from build123d import *

# Parameters (mm, degrees)
SKETCH1_R           = 2.95
SKETCH1_R_2         = 20
SKETCH1_R_3         = 18.5
BOSS_EXTRUDE1_DEPTH = 6
CUT_EXTRUDE2_DEPTH  = 76.689323992
SKETCH4_W           = 6.2
SKETCH4_H           = 2.2
CUT_EXTRUDE3_DEPTH  = 76.689323992


with BuildPart() as part:
    # Sketch1 → Boss-Extrude1 (new body)
    with BuildSketch(Plane.XY):
        Polygon((-32.5, 7.5), (-32.5, -22), (32.5, -22), (32.5, 7.5), (49.675685802, 7.5), (49.675685802, 56.790844389), (-49.675685802, 56.790844389), (-49.675685802, 7.5), align=None)
        Circle(SKETCH1_R, mode=Mode.SUBTRACT)
        with Locations((26.675685802, 31.790844389)):
            Circle(SKETCH1_R_2, mode=Mode.SUBTRACT)
        with Locations((-26.675685802, 31.790844389)):
            Circle(SKETCH1_R_3, mode=Mode.SUBTRACT)
    extrude(amount=BOSS_EXTRUDE1_DEPTH)

    # Sketch3 → Cut-Extrude2 (cut, through all)
    with BuildSketch(Plane.XY.offset(6)):
        Polygon((-12.3, -22), (-7.7, -22), (-7.7, -17), (-5.4, -17), (-5.4, -14), (-7.7, -14), (-7.7, -10), (-12.3, -10), (-12.3, -14), (-14.6, -14), (-14.6, -17), (-12.3, -17), align=None)
        Polygon((7.7, -14), (7.7, -10), (12.3, -10), (12.3, -14), (14.6, -14), (14.6, -17), (12.3, -17), (12.3, -22), (7.7, -22), (7.7, -17), (5.4, -17), (5.4, -14), align=None)
    extrude(amount=-CUT_EXTRUDE2_DEPTH, mode=Mode.SUBTRACT)

    # Sketch4 → Cut-Extrude3 (cut, through all)
    with BuildSketch(Plane.XY.offset(6)):
        with Locations((0, 52.690844389)):
            Rectangle(SKETCH4_W, SKETCH4_H)
        with Locations((44, 52.690844389)):
            Rectangle(SKETCH4_W, SKETCH4_H)
        with Locations((-44, 52.690844389)):
            Rectangle(SKETCH4_W, SKETCH4_H)
    extrude(amount=-CUT_EXTRUDE3_DEPTH, mode=Mode.SUBTRACT)


solid = part.part
Read the model definition and answer for the solid it produces. Units are mm, in the model's axes. A direction names the side the tool comes from. Round coordinates to 2 decimals unless told otherwise and drop trailing zeros. Order: outer loops, then holes, each group sorted by start corner. A loop starts at its lowest first (then second) coordinate and runs counter-clockwise, first axis right, second up.
1) Flat-ended cylindrical pins translate along their axes: pin 1 (1.5 mm diameter, centred on y = -20.5, z = 2.5, fed in from -X); pin 2 (3 mm diameter, centred on y = -12.5, z = 2, fed in from +X); pin 3 (22 mm diameter, centred on x = -26.68, y = 31.79, fed in from +Z). Find the tip coordinate at first contact, or state that the pin passes through.
2) The part is cut by section C-C on y = 49. Write down the section's boundary in (x, z).
3) The mould has two halves that part along Y. Classify faces 4 (the face through (0, 51.591, 3)), 5 (the face through (-7.7, -20, 3)), 6 (the face through (-23, -22, 3)), 7 (the face through (-14.6, -15, 3)): released by +Y, released by -Y, zero draft, split by the parting line, or undercut.
4) The part is cut by section D-D on x = -18.5. Write down the section's boundary in (y, z), plus the area to 3 significant figures.
5) Straight lines are drawn through the part: L1, parallel to X at y = -13, z = 4; L2, parallel to Y at x = 0, z = 2.8; L3, parallel to Y at x = -43.5, z = 4.2. For each, find the intervals that lie inside material, in ascending order.
6) For faces 1 (the face through (-1, 18, 0)), 2 (the face through (-44, 51.591, 3)), 3 (the face through (-12.3, -12, 3)), determine the directions among +Z, -Z, +X, -X, +Y, -Y from which every point of the face is accessible in a straight line to the end or side of a thin tool.
7) The part is cut by section B-B on x = 0. Write down the section's boundary in (y, z), plus the area to 3 significant figures.
8) The part is cut by section A-A on y = 0. Write down the section's boundary in (x, z), plus the area to 3 significant figures.
Resolved:
1. pin 1: stops at x = -32.5
1. pin 2: stops at x = 32.5
1. pin 3: passes through
2. outline: (-49.68, 0) - (-33.47, 0) - (-33.47, 6) - (-49.68, 6) - close; (-19.89, 0) - (16.49, 0) - (16.49, 6) - (-19.89, 6) - close; (36.87, 0) - (49.68, 0) - (49.68, 6) - (36.87, 6) - close
3. face 4: undercut
3. face 5: zero draft
3. face 6: released by -Y
3. face 7: undercut
4. outline: (-22, 0) - (15.2, 0) - (15.2, 6) - (-22, 6) - close; (48.39, 0) - (56.79, 0) - (56.79, 6) - (48.39, 6) - close
4. area: 274 mm2
5. L1: x = -32.5 to -12.3, -7.7 to 7.7, 12.3 to 32.5
5. L2: y = -22 to -2.95, 2.95 to 51.59, 53.79 to 56.79
5. L3: y = 7.5 to 24.1, 39.48 to 51.59, 53.79 to 56.79
6. face 1: -Z, +X, -X, +Y, -Y
6. face 2: +Z, -Z
6. face 3: +Z, -Z, -Y
7. outline: (-22, 0) - (-2.95, 0) - (-2.95, 6) - (-22, 6) - close; (2.95, 0) - (51.59, 0) - (51.59, 6) - (2.95, 6) - close; (53.79, 0) - (56.79, 0) - (56.79, 6) - (53.79, 6) - close
7. area: 424 mm2
8. outline: (-32.5, 0) - (-2.95, 0) - (-2.95, 6) - (-32.5, 6) - close; (2.95, 0) - (32.5, 0) - (32.5, 6) - (2.95, 6) - close
8. area: 355 mm2
